Part model, mm, in its own coordinate system. A direction names the side the tool comes from. Give positions to 0.01 mm unless a question says otherwise; leave off trailing zeros. Order: outer loops, then holes, each group sorted by start corner. A loop starts at its lowest first (then second) coordinate and runs counter-clockwise, first axis right, second up. Notation, with made-up numbers: (73, 55.5) -> (120, 55.5) arc R33 ccw to (120, 94.5) -> close; hole circle Ø8 at (80.5, 26.5). An arc over 180 degrees is marked (long way). Write item = value, one per line. Start each with the question number.
(1) Two-plate mould, pull along Z, no slides. Class faces 1 (the cylindrical face through (23.01, -25.99, -1.23)), 2 (the cylindrical face through (-35.12, -22.48, 7.87)), 3 (the cylindrical face through (34.79, 22.48, 7.3)), 4 (the flat face through (-39.489, -0.42, 15.437)): pulls with the +Z half, pulls with the -Z half, needs draft (parallel to the pull), parting line crosses it, or undercut.
(2) Flat gauge pins, fed straight in: pin 1 (1.5 mm diameter, centred on y = -18.5, z = 8, fed in from -X); pin 2 (6 mm diameter, centred on y = -4.5, z = 9.5, fed in from +X); pin 3 (17 mm diameter, centred on x = -4, y = 1, fed in from +Z); pin 4 (6 mm diameter, centred on x = -2.5, y = 23, fed in from +Z). Where does each tip first touch, or does it go through?
(3) Saw through at A-A, the plane y = 16. List the corners of the cut face in (x, z).
(4) Saw through at B-B, the plane x = -23.55. List the corners of the cut face in (y, z), then the cut area to 3 significant figures.
(5) Which spindle directions (+Z, -Z, +X, -X, +Y, -Y) get a long thin tool onto all of the face, cutting with end or side? Do faces 5 (the flat face through (0, -30, -1)), 6 (the flat face through (33.795, -0.42, 8.109)). Say none if no direction does.
(6) Probe line 1 along Y through (x, z) = (-23.55, -0.7); line 2 along Y through (x, z) = (33, 6.25); line 3 along Z through (x, y) = (-14, -18). List the from-to ranges inside material, lowest first. Write a range as from..to.
(7) Saw through at D-D, the plane y = -23.55. List the corners of the cut face in (x, z).
(8) Saw through at C-C, the plane x = 0. List the corners of the cut face in (y, z).
from build123d import *

# Parameters (mm, degrees)
SCHIZZO1_W               = 64
SCHIZZO1_H               = 60
BASE_FLANGIA1_DEPTH      = 2.5
BORDO_FLANGIA1_START     = -30
BORDO_FLANGIA1_DEPTH     = 60
BORDO_FLANGIA1_2_DEPTH   = 60
BORDO_FLANGIA2_START     = -30
BORDO_FLANGIA2_DEPTH     = 60
BORDO_FLANGIA2_2_DEPTH   = 60
SCHIZZO12_R              = 2.5
SCHIZZO12_R_2            = 20
TAGLIO_ESTRUSIONE1_DEPTH = 10
SCHIZZO14_R              = 2.5
TAGLIO_ESTRUSIONE2_DEPTH = 10


# Read off the part's stored shape, not the designer's step: Bordo-Flangia1, Bordo-Flangia2
# Sheet-metal steps are written as plain solids
with BuildPart() as part:
    # Schizzo1 → Base-Flangia1 (new body)
    with BuildSketch(Plane.XY):
        Rectangle(SCHIZZO1_W, SCHIZZO1_H)
    extrude(amount=-BASE_FLANGIA1_DEPTH)

    # Bordo-Flangia1 outline → Bordo-Flangia1 (cut)
    with BuildSketch(Plane(origin=(0, 0, 0), x_dir=(1, 0, 0), z_dir=(0, 1, 0)).offset(BORDO_FLANGIA1_START)):
        with BuildLine():
            ThreePointArc((28.687972446, 2.5), (30.306272446, 2.066377822), (31.490950268, 0.8817))
            Line((31.490950268, 0.8817), (32, 0))
            Line((32, 0), (32, 2.5))
            Line((32, 2.5), (28.687972446, 2.5))
        make_face()
    extrude(amount=BORDO_FLANGIA1_DEPTH, mode=Mode.SUBTRACT)

    # Bordo-Flangia1 2 outline → Bordo-Flangia1 2 (add)
    with BuildSketch(Plane(origin=(0, 0, 0), x_dir=(1, 0, 0), z_dir=(0, 1, 0)).offset(BORDO_FLANGIA1_START)):
        with BuildLine():
            Line((40.556624327, -14.820508076), (32, 0))
            Line((32, 0), (28.687972446, 0))
            ThreePointArc((28.687972446, 0), (29.056272446, -0.098685688), (29.325886758, -0.3683))
            Line((29.325886758, -0.3683), (38.391560818, -16.070508076))
            Line((38.391560818, -16.070508076), (40.556624327, -14.820508076))
        make_face()
    extrude(amount=BORDO_FLANGIA1_2_DEPTH)

    # Bordo-Flangia2 outline → Bordo-Flangia2 (cut)
    with BuildSketch(Plane(origin=(0, 0, 0), x_dir=(1, 0, 0), z_dir=(0, 1, 0)).offset(BORDO_FLANGIA2_START)):
        with BuildLine():
            Line((-32, 0), (-31.490950268, 0.8817))
            ThreePointArc((-31.490950268, 0.8817), (-30.306272446, 2.066377822), (-28.687972446, 2.5))
            Line((-28.687972446, 2.5), (-32, 2.5))
            Line((-32, 2.5), (-32, 0))
        make_face()
    extrude(amount=BORDO_FLANGIA2_DEPTH, mode=Mode.SUBTRACT)

    # Bordo-Flangia2 2 outline → Bordo-Flangia2 2 (add)
    with BuildSketch(Plane(origin=(0, 0, 0), x_dir=(1, 0, 0), z_dir=(0, 1, 0)).offset(BORDO_FLANGIA2_START)):
        with BuildLine():
            Line((-28.687972446, 0), (-32, 0))
            Line((-32, 0), (-40.556624327, -14.820508076))
            Line((-40.556624327, -14.820508076), (-38.391560818, -16.070508076))
            Line((-38.391560818, -16.070508076), (-29.325886758, -0.3683))
            ThreePointArc((-29.325886758, -0.3683), (-29.056272446, -0.098685688), (-28.687972446, 0))
        make_face()
    extrude(amount=BORDO_FLANGIA2_2_DEPTH)

    # Schizzo12 → Taglio-Estrusione1 (cut)
    with BuildSketch(Plane.XY):
        with Locations((-23.55, 23.55)):
            Circle(SCHIZZO12_R)
        with Locations((23.55, 23.55)):
            Circle(SCHIZZO12_R)
        with Locations((23.55, -23.55)):
            Circle(SCHIZZO12_R)
        with Locations((-23.55, -23.55)):
            Circle(SCHIZZO12_R)
        Circle(SCHIZZO12_R_2)
    extrude(amount=-TAGLIO_ESTRUSIONE1_DEPTH, mode=Mode.SUBTRACT)

    # Schizzo14 → Taglio-Estrusione2 (cut)
    with BuildSketch(Plane(origin=(-24, 0, -13.856406461), x_dir=(-0.5000000000000043, 0, 0.8660254037844363), z_dir=(-0.8660254037844362, 0, -0.5000000000000042))):
        with Locations((24.047574595, 20)):
            Circle(SCHIZZO14_R)
        with Locations(Location((24.047574595, -20, 0), (0, 0, 180))):
            Circle(SCHIZZO14_R)
    taglio_estrusione2 = extrude(amount=-TAGLIO_ESTRUSIONE2_DEPTH, mode=Mode.SUBTRACT)

    # Specchia1: Taglio-Estrusione2 across plane
    add(taglio_estrusione2.mirror(Plane(origin=(0, 0, 0), x_dir=(0, 0, 1), z_dir=(1, 0, 0))), mode=Mode.SUBTRACT)


solid = part.part
Results list:
q1.face_1 = needs draft
q1.face_2 = undercut
q1.face_3 = undercut
q1.face_4 = pulls with the +Z half
q2.pin_1 = -37.05
q2.pin_2 = 39.22
q2.pin_3 = through
q2.pin_4 = 0
q3.outline = (-40.56, 14.82) -> (-31.49, -0.88) arc R3.24 ccw to (-28.69, -2.5) -> (-12, -2.5) -> (-12, 0) -> (-28.69, 0) arc R0.74 cw to (-29.33, 0.37) -> (-38.39, 16.07) -> close; (12, -2.5) -> (28.69, -2.5) arc R3.24 ccw to (31.49, -0.88) -> (40.56, 14.82) -> (38.39, 16.07) -> (29.33, 0.37) arc R0.74 cw to (28.69, 0) -> (12, 0) -> close
q4.outline = (-30, -2.5) -> (-26.05, -2.5) -> (-26.05, 0) -> (-30, 0) -> close; (-21.05, -2.5) -> (21.05, -2.5) -> (21.05, 0) -> (-21.05, 0) -> close; (26.05, -2.5) -> (30, -2.5) -> (30, 0) -> (26.05, 0) -> close
q4.area = 125 mm^2
q5.face_5 = +Z, -Z, +X, -X, -Y
q5.face_6 = +Z, +Y, -Y
q6.line_1 = -30..-26.05, -21.05..21.05, 26.05..30
q6.line_2 = -30..-21.3, -18.7..18.7, 21.3..30
q6.line_3 = -2.5..0
q7.outline = (-40.56, 14.82) -> (-31.49, -0.88) arc R3.24 ccw to (-28.69, -2.5) -> (-26.05, -2.5) -> (-26.05, 0) -> (-28.69, 0) arc R0.74 cw to (-29.33, 0.37) -> (-38.39, 16.07) -> close; (-21.05, -2.5) -> (21.05, -2.5) -> (21.05, 0) -> (-21.05, 0) -> close; (26.05, -2.5) -> (28.69, -2.5) arc R3.24 ccw to (31.49, -0.88) -> (40.56, 14.82) -> (38.39, 16.07) -> (29.33, 0.37) arc R0.74 cw to (28.69, 0) -> (26.05, 0) -> close
q8.outline = (-30, -2.5) -> (-20, -2.5) -> (-20, 0) -> (-30, 0) -> close; (20, -2.5) -> (30, -2.5) -> (30, 0) -> (20, 0) -> close
